CAD build for the part. Positions are in the model's coordinates, mm. Face numbers are marked on the shaded views. A direction names the side the tool comes from. Give positions to 0.01 mm unless a question says otherwise; leave off trailing zeros. Order: outer loops, then holes, each group sorted by start corner. A loop starts at its lowest first (then second) coordinate and runs counter-clockwise, first axis right, second up.
Item 1: Which spindle directions (+Z, -Z, +X, -X, +Y, -Y) get a long thin tool onto all of the face, cutting with end or side? Do the marked faces 4 and 5. Say none if no direction does.
Item 2: Band-saw the part on B-B on y = 0. Give the cut face in (x, z), plus the area to 3 significant figures.
Item 3: Two-plate mould, pull along Z, no slides. Class the marked faces 1, 2 and 3: released by +Z, released by -Z, zero draft, split by the parting line, or undercut.
Item 4: Wall check: L1, parallel to Y at x = 8, z = 0; L2, parallel to Z at x = 12.25, y = 13; L3, parallel to Z at x = 10.75, y = 11. Give the ranges that are in metal, low to high.
Item 5: Band-saw the part on C-C on x = 6.5. Give the cut face in (y, z).
Item 6: Band-saw the part on D-D on x = 2. Give the cut face in (y, z), plus the area to 3 significant figures.
Item 7: Flat gauge pins, fed straight in: P1, Ø5.5, axis at y = -17.5, z = -6, coming from the +X side; P2, Ø4, axis at y = -15.75, z = 0, coming from the +X side; P3, Ø2, axis at x = 5, z = -19.5, coming from the +Y side; P4, Ø4, axis at y = -11.14, z = 11.14, coming from the +X side. Where does each tip first touch, or does it go through?
Item 8: Band-saw the part on A-A on z = 0. Give the cut face in (x, y).
```python
from build123d import *

# Parameters (mm, degrees)
SKETCH1_W                      = 2.5
SKETCH1_H                      = 30
SKETCH2_R                      = 25
BOSS_EXTRUDE1_DEPTH            = 10
CUT_EXTRUDE1_DEPTH             = 0.5
CUT_EXTRUDE2_DEPTH             = 0.5
CUT_EXTRUDE3_DEPTH             = 0.5
F_12_0_12_DIAMETER_HOLE1_D     = 12
F_12_0_12_DIAMETER_HOLE1_DEPTH = 12.5
F_7_0_7_DIAMETER_HOLE1_D       = 7
F_7_0_7_DIAMETER_HOLE1_DEPTH   = 0.5
F_4_2_4_2_DIAMETER_HOLE1_D     = 4.2
F_4_2_4_2_DIAMETER_HOLE1_DEPTH = 12.5
F_5_0_5_DIAMETER_HOLE1_D       = 5
F_5_0_5_DIAMETER_HOLE1_DEPTH   = 7
CHAMFER1_SIZE                  = 0.5


with BuildPart() as part:
    # Sketch1 → Revolve1 (revolve)
    with BuildSketch(Plane.XY):
        with Locations((11.25, 15)):
            Rectangle(SKETCH1_W, SKETCH1_H)
    revolve(axis=Axis((10, 0, 0), (1, 0, 0)))

    # Sketch2 → Boss-Extrude1 (add)
    with BuildSketch(Plane.ZY.offset(-10)):
        Circle(SKETCH2_R)
    extrude(amount=BOSS_EXTRUDE1_DEPTH)

    # Sketch3 → Cut-Extrude1 (cut)
    with BuildSketch(Plane(origin=(12.5, 0, 0), x_dir=(0, 0, -1), z_dir=(1, 0, 0))):
        with BuildLine():
            ThreePointArc((13.396253221, 5.548909769), (14.5, 0), (13.396253221, -5.548909769))
            ThreePointArc((13.396253221, -5.548909769), (15.290439572, -10.121880146), (19.863409949, -8.227693796))
            ThreePointArc((19.863409949, -8.227693796), (21.5, 0), (19.863409949, 8.227693796))
            ThreePointArc((19.863409949, 8.227693796), (15.290439572, 10.121880146), (13.396253221, 5.548909769))
        make_face()
    extrude(amount=-CUT_EXTRUDE1_DEPTH, mode=Mode.SUBTRACT)

    # Sketch4 → Cut-Extrude2 (cut)
    with BuildSketch(Plane(origin=(12.5, 0, 0), x_dir=(0, 0, -1), z_dir=(1, 0, 0))):
        with BuildLine():
            ThreePointArc((-5.548909769, 13.396253221), (0, 14.5), (5.548909769, 13.396253221))
            ThreePointArc((5.548909769, 13.396253221), (10.121880146, 15.290439572), (8.227693796, 19.863409949))
            ThreePointArc((8.227693796, 19.863409949), (0, 21.5), (-8.227693796, 19.863409949))
            ThreePointArc((-8.227693796, 19.863409949), (-10.121880146, 15.290439572), (-5.548909769, 13.396253221))
        make_face()
    extrude(amount=-CUT_EXTRUDE2_DEPTH, mode=Mode.SUBTRACT)

    # Sketch5 → Cut-Extrude3 (cut)
    with BuildSketch(Plane(origin=(12.5, 0, 0), x_dir=(0, 0, -1), z_dir=(1, 0, 0))):
        with BuildLine():
            ThreePointArc((-13.396253221, -5.548909769), (-14.5, 0), (-13.396253221, 5.548909769))
            ThreePointArc((-13.396253221, 5.548909769), (-15.290439572, 10.121880146), (-19.863409949, 8.227693796))
            ThreePointArc((-19.863409949, 8.227693796), (-21.5, 0), (-19.863409949, -8.227693796))
            ThreePointArc((-19.863409949, -8.227693796), (-15.290439572, -10.121880146), (-13.396253221, -5.548909769))
        make_face()
    extrude(amount=-CUT_EXTRUDE3_DEPTH, mode=Mode.SUBTRACT)

    # Ø12.0 (12) Diameter Hole1
    with Locations(Plane.ZY):
        with Locations((0, 0)):
            Hole(F_12_0_12_DIAMETER_HOLE1_D / 2, depth=F_12_0_12_DIAMETER_HOLE1_DEPTH)

    # Ø7.0 (7) Diameter Hole1
    with Locations(Plane(origin=(12.5, 0, 0), x_dir=(0, 0, -1), z_dir=(1, 0, 0))):
        with Locations((-6.888301783, -16.629831585), (6.888301783, -16.629831585)):
            Hole(F_7_0_7_DIAMETER_HOLE1_D / 2, depth=F_7_0_7_DIAMETER_HOLE1_DEPTH)

    # Ø4.2 (4.2) Diameter Hole1
    with Locations(Plane.ZY):
        with Locations((-11.136931804, -11.136931804), (-11.136931804, 11.136931804), (11.136931804, 11.136931804), (11.136931804, -11.136931804)):
            Hole(F_4_2_4_2_DIAMETER_HOLE1_D / 2, depth=F_4_2_4_2_DIAMETER_HOLE1_DEPTH)

    # Ø5.0 (5) Diameter Hole1
    with Locations(Plane(origin=(12.5, 0, 0), x_dir=(0, 0, -1), z_dir=(1, 0, 0))):
        with Locations((0, -15.75)):
            Hole(F_5_0_5_DIAMETER_HOLE1_D / 2, depth=F_5_0_5_DIAMETER_HOLE1_DEPTH)

    # Chamfer1
    chamfer1_edges = [part.edges().sort_by_distance(p)[0] for p in [
        (12.5, -30, 0),
    ]]
    chamfer(chamfer1_edges, length=CHAMFER1_SIZE)


solid = part.part
```
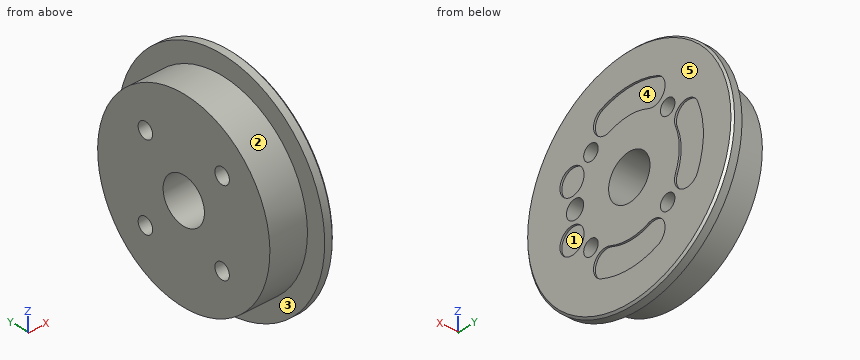
The answers:
1. face 4: +X
1. face 5: +Z, -Z, +X, +Y, -Y
2. outline: (0, -25) - (10, -25) - (10, -30) - (12, -30) - (12.5, -29.5) - (12.5, -21.5) - (12, -21.5) - (12, -14.5) - (12.5, -14.5) - (12.5, -6) - (0, -6) - close; (0, 6) - (12.5, 6) - (12.5, 14.5) - (12, 14.5) - (12, 21.5) - (12.5, 21.5) - (12.5, 29.5) - (12, 30) - (10, 30) - (10, 25) - (0, 25) - close
2. area: 493 mm2
3. face 1: undercut
3. face 2: split by the parting line
3. face 3: zero draft
4. L1: y = -25 to -18.25, -13.25 to -6, 6 to 25
4. L2: z = -26.76 to -12.11, -10.17 to 10.17, 12.11 to 26.76
4. L3: z = -27.91 to -13.23, -9.04 to 9.04, 13.23 to 27.91
5. outline: circle Ø50 at (0, 0); hole circle Ø5 at (-15.75, 0); hole circle Ø4.2 at (-11.14, -11.14); hole circle Ø4.2 at (-11.14, 11.14); hole circle Ø12 at (0, 0); hole circle Ø4.2 at (11.14, -11.14); hole circle Ø4.2 at (11.14, 11.14)
6. outline: circle Ø50 at (0, 0); hole circle Ø4.2 at (-11.14, -11.14); hole circle Ø4.2 at (-11.14, 11.14); hole circle Ø12 at (0, 0); hole circle Ø4.2 at (11.14, -11.14); hole circle Ø4.2 at (11.14, 11.14)
6. area: 1,790 mm2
7. P1: stops at x = 12.5
7. P2: stops at x = 5.5
7. P3: stops at y = 16.82
7. P4: passes through
8. outline: (0, -25) - (10, -25) - (10, -30) - (12, -30) - (12.5, -29.5) - (12.5, -18.25) - (5.5, -18.25) - (5.5, -13.25) - (12.5, -13.25) - (12.5, -6) - (0, -6) - close; (0, 6) - (12.5, 6) - (12.5, 14.5) - (12, 14.5) - (12, 21.5) - (12.5, 21.5) - (12.5, 29.5) - (12, 30) - (10, 30) - (10, 25) - (0, 25) - close
